The model under review builds one solid part; all positions refer to its coordinate system, in mm. Face numbers are marked on the shaded views. A direction names the side the tool comes from. Give positions to 0.01 mm unless a question says otherwise; leave off trailing zeros. Order: outer loops, then holes, each group sorted by start corner. A loop starts at its lowest first (then second) coordinate and runs counter-clockwise, first axis right, second up.
```python
from build123d import *

# Parameters (mm, degrees)
F1_DEPTH = 63.5
F0_W     = 25.298796773
F0_H     = 19.05
F2_DEPTH = 25.4
F3_DEPTH = 7.9375


with BuildPart() as f1:
    # F0 (on Front) → F1 (new body, symmetric)
    with BuildSketch(Plane.XZ):
        Polygon((-41.275, -9.525), (41.275, -9.525), (41.275, 9.525), (22.225, 9.525), (-41.275, 9.525), align=None)
    extrude(amount=F1_DEPTH, both=True)

    # F0 (on Front) → F2 (join, symmetric)
    with BuildSketch(Plane.XZ):
        with BuildLine():
            Line((22.225, 9.525), (41.275, 9.525))
            Line((41.275, 9.525), (41.275, 27.0002))
            ThreePointArc((41.275, 27.0002), (45.9246798487, 38.2255201513), (57.15, 42.8752))
            Line((57.15, 42.8752), (60.426203227, 42.8752))
            Line((60.426203227, 42.8752), (60.426203227, 61.9252))
            Line((60.426203227, 61.9252), (57.15, 61.9252))
            add(Edge.make_bspline(
                [(56.6191061184, 61.9211647159), (56.7959952463, 61.9227867022), (56.9729603774, 61.9241320768), (57.15, 61.9252)],
                knots=[111.1292180124, 111.1292180124, 111.1292180124, 111.1292180124, 111.5045361635, 111.5045361635, 111.5045361635, 111.5045361635], degree=3))
            ThreePointArc((56.6191061184, 61.9211647159), (32.2673042677, 51.5074862246), (22.225, 27.0002))
            Line((22.225, 27.0002), (22.225, 9.525))
        make_face()
        with Locations((73.0756016135, 52.4002)):
            Rectangle(F0_W, F0_H)
    extrude(amount=F2_DEPTH, both=True)

    # F0 (on Front) → F3 (join, symmetric)
    with BuildSketch(Plane.XZ):
        with BuildLine():
            add(Edge.make_bspline(
                [(-41.275, 9.525), (-41.4689858788, 36.7097428775), (4.2434072851, 61.440905318), (56.6191061184, 61.9211647159)],
                knots=[0, 0, 0, 0, 111.1292180124, 111.1292180124, 111.1292180124, 111.1292180124], degree=3))
            Line((-41.275, 9.525), (22.225, 9.525))
            Line((22.225, 9.525), (22.225, 27.0002))
            ThreePointArc((22.225, 27.0002), (32.2673042677, 51.5074862246), (56.6191061184, 61.9211647159))
        make_face()
    extrude(amount=F3_DEPTH, both=True)

    # F0 (on Front) → F4 (revolve)
    with BuildSketch(Plane.XZ):
        Polygon((85.826203227, 66.675), (85.725, 38.1), (111.226203227, 38.1), (111.226203227, 66.675), align=None)
    revolve(axis=Axis((85.7756016135, 0, 52.3875), (-0.003541648, 0, -0.9999937283)))


solid = f1.part
```
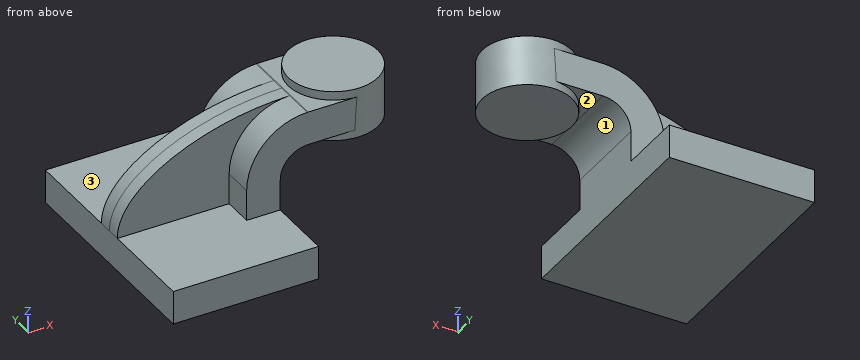
Item 1: Take a section at B-B (z = -4.5). Give the boundary of the cut face in (x, y) (3 decimals).
Values found:
outline: (-41.275, -63.5) - (41.275, -63.5) - (41.275, 63.5) - (-41.275, 63.5) - close
Item 2: Clearance check with flat-ended pins moving along their axes: pin 1 Ø8 at (y, z) = (28.5, 56.5) entering from -X; pin 2 Ø21 at (x, y) = (71.5, -11) entering from -Z; pin 3 Ø10 at (y, z) = (34, 12.5) entering from -X (3 decimals); pin 4 Ø5 at (x, y) = (-22, 42.5) entering from +Z (3 decimals). State where each tip first meets the part, or that it passes through.
Values found:
pin 1: stops at x = 34.96
pin 2: stops at z = 38.15
pin 3: stops at x = -41.275
pin 4: stops at z = 9.525
Item 3: For the marked faces 1, 2 and 3, list the 3-axis set-ups (+Z, -Z, +X, -X, +Y, -Y) from which the entire face can be reached by the end or side of a thin tool; tool diameter is ignored.
Values found:
face 1: -Z, +Y, -Y
face 2: -Z
face 3: +Z, -X, +Y
Item 4: For line 1 (Y direction, x = -15.5, z = 32.5); line 2 (X direction, y = -48, z = 9) (3 decimals); line 3 (X direction, y = -18, z = 22) (3 decimals), list the stretches that pass through material, from the lowest coordinate up.
Values found:
line 1: y = -7.94 to 7.94
line 2: x = -41.275 to 41.275
line 3: x = 22.225 to 41.275
Item 5: Take a section at A-A (y = 38.5). Give the boundary of the cut face in (x, z) (3 decimals).
Values found:
outline: (-41.275, -9.525) - (41.275, -9.525) - (41.275, 9.525) - (-41.275, 9.525) - close
